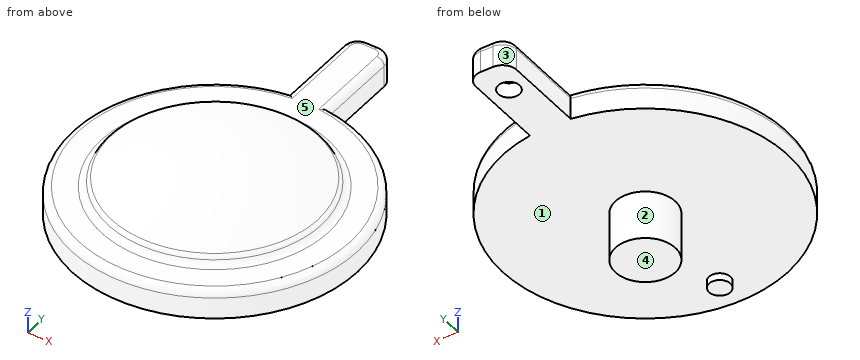
from build123d import *

# Parameters (mm, degrees)
ESQUISSE1_R             = 20
BOSS_EXTRU_1_DEPTH      = 4
ESQUISSE4_R             = 4
BOSS_EXTRU_3_DEPTH      = 6.843
BOSS_EXTRU_4_DEPTH      = 4
ESQUISSE6_R             = 1.5
ENL_V_MAT_EXTRU_1_DEPTH = 2.1
ESQUISSE7_R             = 1.5
BOSS_EXTRU_5_DEPTH      = 1
ESQUISSE8_R             = 4.2
BOSS_EXTRU_6_DEPTH      = 6.843
ESQUISSE9_R             = 14.967417913
BOSS_EXTRU_7_DEPTH      = 1
D_ME1_FACE_RADIUS       = 14.967417913
D_ME1_HEIGHT            = 4
CONG_1_R                = 1
CONG_2_R                = 1
CONG_3_R                = 1


with BuildPart() as part:
    # Esquisse1 → Boss.-Extru.1 (new body)
    with BuildSketch(Plane.XY):
        Circle(ESQUISSE1_R)
    extrude(amount=BOSS_EXTRU_1_DEPTH)

    # Esquisse4 → Boss.-Extru.3 (add)
    with BuildSketch(Plane(origin=(0, 0, 0), x_dir=(-1, 0, 0), z_dir=(0, 0, -1))):
        with Locations(Location((0, 0, 0), (0, 0, 180))):
            Circle(ESQUISSE4_R)
    extrude(amount=BOSS_EXTRU_3_DEPTH)

    # Esquisse5 → Boss.-Extru.4 (add)
    with BuildSketch(Plane(origin=(0, 0, 0), x_dir=(-1, 0, 0), z_dir=(0, 0, -1))):
        with BuildLine():
            Line((2.858287427, 14.40822907), (-2.858287427, 14.40822907))
            Line((-2.858287427, 14.40822907), (-2.858287427, 31.050344996))
            ThreePointArc((-2.858287427, 31.050344996), (-2.27250099, 32.464558559), (-0.858287427, 33.050344996))
            Line((-0.858287427, 33.050344996), (0.858287427, 33.050344996))
            ThreePointArc((0.858287427, 33.050344996), (2.27250099, 32.464558559), (2.858287427, 31.050344996))
            Line((2.858287427, 31.050344996), (2.858287427, 14.40822907))
        make_face()
    extrude(amount=-BOSS_EXTRU_4_DEPTH)

    # Esquisse6 → Enlèv. mat.-Extru.1 (cut)
    with BuildSketch(Plane(origin=(0, 0, 0), x_dir=(-1, 0, 0), z_dir=(0, 0, -1))):
        with Locations((0, 28.410842354)):
            Circle(ESQUISSE6_R)
    extrude(amount=-ENL_V_MAT_EXTRU_1_DEPTH, mode=Mode.SUBTRACT)

    # Esquisse7 → Boss.-Extru.5 (add)
    with BuildSketch(Plane(origin=(0, 0, 0), x_dir=(-1, 0, 0), z_dir=(0, 0, -1))):
        with Locations(Location((0, -15.504004846, 0), (0, 0, 180))):
            Circle(ESQUISSE7_R)
    extrude(amount=BOSS_EXTRU_5_DEPTH)

    # Esquisse8 → Boss.-Extru.6 (add)
    with BuildSketch(Plane(origin=(0, 0, 0), x_dir=(-1, 0, 0), z_dir=(0, 0, -1))):
        with Locations(Location((0, 0, 0), (0, 0, 180))):
            Circle(ESQUISSE8_R)
    extrude(amount=BOSS_EXTRU_6_DEPTH)

    # Esquisse9 → Boss.-Extru.7 (add)
    with BuildSketch(Plane.XY.offset(4)):
        Circle(ESQUISSE9_R)
    extrude(amount=BOSS_EXTRU_7_DEPTH)

    # Dôme1: a dome of height H over a round flat face of radius A is a cap of a sphere of radius (A * A + H * H) / (2 * H)
    d_me1_r = (D_ME1_FACE_RADIUS * D_ME1_FACE_RADIUS + D_ME1_HEIGHT * D_ME1_HEIGHT) / (2 * D_ME1_HEIGHT)
    d_me1_base = Plane((0, 0, 5), z_dir=(0, 0, 1))
    with Locations(d_me1_base.offset(D_ME1_HEIGHT - d_me1_r)):
        d_me1_ball = Sphere(d_me1_r, mode=Mode.PRIVATE)
    add(split(d_me1_ball, bisect_by=d_me1_base, keep=Keep.TOP, mode=Mode.PRIVATE))

    # Congé1
    cong_1_edges = [part.edges().sort_by_distance(p)[0] for p in [
        (-14.967417913, 0, 5),
    ]]
    fillet(cong_1_edges, radius=CONG_1_R)

    # Congé2
    cong_2_edges = [part.edges().sort_by_distance(p)[0] for p in [
        (-14.967417913, 0, 4),
    ]]
    fillet(cong_2_edges, radius=CONG_2_R)

    # Congé3
    cong_3_edges = [part.edges().sort_by_distance(p)[0] for p in [
        (0, -20, 4),
        (-2.858287427, 25.422523065, 4),
        (2.858287427, 25.422523065, 4),
        (2.27250099, 32.464558559, 4),
        (0, 33.050344996, 4),
        (-2.27250099, 32.464558559, 4),
    ]]
    fillet(cong_3_edges, radius=CONG_3_R)


solid = part.part
Read the model definition and answer for the solid it produces. Units are mm, in the model's axes. Face numbers are marked on the shaded views. A direction names the side the tool comes from. Coordinates: 2 decimals unless noted, no trailing zeros. Loops run counter-clockwise (first coordinate to the right, second up) from the corner with the lowest first, then second, coordinate; pieces in that order, holes last. Notation, with made-up numbers: (89.5, 81.5) -> (135.5, 81.5) arc R15 ccw to (135.5, 92.5) -> close; hole circle Ø6 at (-27.5, 74.5). An arc over 180 degrees is marked (long way). Write item = value, one per line. Start each with the question number.
1) Find the intervals of material crossed by L1, parallel to Z at x = 2, y = 17; L2, parallel to X at y = 8.5, z = 5; L3, parallel to Z at x = 2.5, y = 30, in increasing order. Write a range as from..to.
2) The part is cut by section B-B, the plane z = -5. Determine the outline of the cut face in (x, y).
3) The part is cut by section A-A, the plane y = 23.5. Determine the outline of the cut face in (x, z), plus the area to 3 significant figures.
4) The part is cut by section D-D, the plane z = 7.25. Determine the outline of the cut face in (x, y).
5) Given P1, Ø2, axis at y = 5.5, z = 6.5, coming from the +X side (3 decimals); P2, Ø2.5, axis at y = 23, z = 1.5, coming from the -X side; P3, Ø2.5, axis at x = 0, y = 28.41, coming from the -Z side; P4, Ø4, axis at x = -10, z = -2.5, coming from the +Y side, each flat-ended and moving along its own axis, determine where each tip first touches the part or whether it passes through.
6) The mould has two halves that part along X. Classify the marked faces 1, 2 and 3: pulls with the +X half, pulls with the -X half, needs draft (parallel to the pull), parting line crosses it, or undercut.
7) The part is cut by section C-C, the plane y = 29. Determine the outline of the cut face in (x, z).
8) For the marked faces 4 and 5, determine the directions among +Z, -Z, +X, -X, +Y, -Y from which every point of the face is accessible in a straight line to the end or side of a thin tool.
Result:
q1.L1 = 0..4
q1.L2 = -12.09..12.09
q1.L3 = 0..3.77
q2.outline = circle Ø8.4 at (0, 0)
q3.outline = (-2.86, 0) -> (2.86, 0) -> (2.86, 3) arc R1 ccw to (1.86, 4) -> (-1.86, 4) arc R1 ccw to (-2.86, 3) -> close
q3.area = 22.4 mm²
q4.outline = circle Ø20.19 at (0, 0)
q5.P1 = 12.985
q5.P2 = -2.86
q5.P3 = 2.1
q5.P4 = through
q6.face_1 = needs draft
q6.face_2 = parting line crosses it
q6.face_3 = pulls with the -X half
q7.outline = (-2.86, 0) -> (-1.38, 0) -> (-1.38, 2.1) -> (1.38, 2.1) -> (1.38, 0) -> (2.86, 0) -> (2.86, 3) arc R1 ccw to (1.86, 4) -> (-1.86, 4) arc R1 ccw to (-2.86, 3) -> close
q8.face_4 = -Z, +X, -X, +Y, -Y
q8.face_5 = +Z
